```python
from build123d import *

# Parameters (mm, degrees)
SKETCH1_W                    = 50
SKETCH1_H                    = 234
BOSS_EXTRUDE1_DEPTH          = 18
F_4_0_4_DIAMETER_HOLE2_D     = 4
F_4_0_4_DIAMETER_HOLE2_DEPTH = 30
F_4_0_4_DIAMETER_HOLE2_TIP   = 1.201721238
F_4_0_4_DIAMETER_HOLE3_D     = 4
F_4_0_4_DIAMETER_HOLE3_DEPTH = 30
F_4_0_4_DIAMETER_HOLE3_TIP   = 1.201721238


with BuildPart() as part:
    # Sketch1 → Boss-Extrude1 (new body)
    with BuildSketch(Plane.XY):
        Rectangle(SKETCH1_W, SKETCH1_H)
    extrude(amount=BOSS_EXTRUDE1_DEPTH)

    # Ø4.0 (4) Diameter Hole2
    with Locations(Plane(origin=(25, 0, 0), x_dir=(0, 0, -1), z_dir=(1, 0, 0))):
        with Locations((-9, 64), (-9, -64)):
            Hole(F_4_0_4_DIAMETER_HOLE2_D / 2, depth=F_4_0_4_DIAMETER_HOLE2_DEPTH)
            with Locations((0, 0, -(F_4_0_4_DIAMETER_HOLE2_DEPTH + F_4_0_4_DIAMETER_HOLE2_TIP / 2))):  # 118° drill point
                Cone(0, F_4_0_4_DIAMETER_HOLE2_D / 2, F_4_0_4_DIAMETER_HOLE2_TIP, mode=Mode.SUBTRACT)

    # Ø4.0 (4) Diameter Hole3
    with Locations(Plane.ZY.offset(25)):
        with Locations((9, 85), (9, 0), (9, -85)):
            Hole(F_4_0_4_DIAMETER_HOLE3_D / 2, depth=F_4_0_4_DIAMETER_HOLE3_DEPTH)
            with Locations((0, 0, -(F_4_0_4_DIAMETER_HOLE3_DEPTH + F_4_0_4_DIAMETER_HOLE3_TIP / 2))):  # 118° drill point
                Cone(0, F_4_0_4_DIAMETER_HOLE3_D / 2, F_4_0_4_DIAMETER_HOLE3_TIP, mode=Mode.SUBTRACT)


solid = part.part
```
Here's how the part is built. I have some questions about the finished solid (model axes, mm). A direction names the side the tool comes from. Give positions to 0.01 mm unless a question says otherwise; leave off trailing zeros. Answer as a JSON object with one key per item and string values. Group by question number.
Item 1: Please list where these lines run through material, in increasing order: probe 1 along Y at (x, z) = (-17, 9.25); probe 2 along Y at (x, z) = (2.75, 9); probe 3 along Z at (x, y) = (-7.5, 0).
Item 2: Which directions (+Z, -Z, +X, -X, +Y, -Y) give clear straight access to the entire face, cutting with the end or side of a thin tool? Please do faces 4 (the cylindrical face through (-9.8, -1.2, 10.6)), 5 (the flat face through (0, 2, 18)), 6 (the cylindrical face through (10, -62, 9)).
Item 3: If we mould it in two halves opening along Z, with no side actions, what happens to faces 1 (the flat face through (0, 2, 0)), 2 (the conical face through (5.99, -0.21, 8.72)), 3 (the flat face through (-25, -2, 11))? For each: pulls with the +Z half, pulls with the -Z half, needs draft (parallel to the pull), parting line crosses it, or undercut.
Item 4: For P1, Ø2.5, axis at y = 64, z = 9, coming from the +X side; P2, Ø8, axis at x = 3, y = -21.5, coming from the -Z side, each with a flat end and sliding along its axis, tell me the tip position at first contact or that it passes through.
Result set:
{
 "1": {"probe 1": "-117 to -86.98, -83.02 to -1.98, 1.98 to 83.02, 86.98 to 117", "probe 2": "-117 to -87, -83 to -66, -62 to -2, 2 to 62, 66 to 83, 87 to 117", "probe 3": "0 to 7, 11 to 18"},
 "2": {"face 4": "-X", "face 5": "+Z, +X, -X, +Y, -Y", "face 6": "+X"},
 "3": {"face 1": "pulls with the -Z half", "face 2": "undercut", "face 3": "needs draft"},
 "4": {"P1": "x = -5.45", "P2": "z = 0"}
}
